CAD build for the part. Positions are in the model's coordinates, mm. A direction names the side the tool comes from. Give positions to 0.01 mm unless a question says otherwise; leave off trailing zeros. Order: outer loops, then holes, each group sorted by start corner. A loop starts at its lowest first (then second) coordinate and runs counter-clockwise, first axis right, second up. Notation, with made-up numbers: (9.25, 21.25) -> (67.25, 21.25) arc R20 cw to (67.25, 42.25) -> close; hole circle Ø4 at (-10, 76.25). An arc over 180 degrees is marked (long way). Answer as CSV lines item,"result".
```python
from build123d import *

# Parameters (mm, degrees)
SKETCH1_R            = 1.25
BOSS_EXTRUDE1_DEPTH  = 2.5
SKETCH3_W            = 12.5
SKETCH3_H            = 28.9
BOSS_EXTRUDE2_DEPTH  = 5.38
CUT_EXTRUDE1_DEPTH   = 9
LPATTERN1_COUNT      = 4
LPATTERN1_PITCH      = 10
LPATTERN1_COUNT_DIR2 = 2
LPATTERN1_PITCH_DIR2 = 10


with BuildPart() as part:
    # Sketch1 → Boss-Extrude1 (new body)
    with BuildSketch(Plane.XY):
        Polygon((9.79, -14.45), (-8.795857864, -14.45), (-10, -14.45), (-10, 14.45), (-9.79, 14.45), (8.795857864, 14.45), (10, 14.45), (10, -14.45), align=None)
        with Locations((-7.5, -5)):
            Circle(SKETCH1_R, mode=Mode.SUBTRACT)
        with Locations((-7.5, 5)):
            Circle(SKETCH1_R, mode=Mode.SUBTRACT)
        with Locations((7.5, 5)):
            Circle(SKETCH1_R, mode=Mode.SUBTRACT)
        with Locations((7.5, -5)):
            Circle(SKETCH1_R, mode=Mode.SUBTRACT)
    extrude(amount=BOSS_EXTRUDE1_DEPTH)

    # Sketch3 → Boss-Extrude2 (add)
    with BuildSketch(Plane.ZY.offset(10)):
        with Locations((-3.75, 0)):
            Rectangle(SKETCH3_W, SKETCH3_H)
    extrude(amount=BOSS_EXTRUDE2_DEPTH)

    # Sketch4 → Cut-Extrude1 (cut)
    with BuildSketch(Plane(origin=(0, 0, -10), x_dir=(-1, 0, 0), z_dir=(0, 0, -1))):
        with BuildLine():
            Line((13.62129958, 14.447528029), (13.62129958, 14.194772629))
            ThreePointArc((13.62129958, 14.194772629), (13.584011291, 14.095850288), (13.49070263, 14.046155824))
            ThreePointArc((13.49070263, 14.046155824), (13.278327951, 13.994947975), (13.081809662, 13.899523608))
            ThreePointArc((13.081809662, 13.899523608), (12.85675958, 13.447530026), (13.081809666, 12.995536447))
            ThreePointArc((13.081809666, 12.995536447), (13.278327608, 12.9001091), (13.490702635, 12.848898474))
            ThreePointArc((13.490702635, 12.848898474), (13.584017776, 12.799196632), (13.62129958, 12.700262029))
            Line((13.62129958, 12.700262029), (13.62129958, 12.194776629))
            ThreePointArc((13.62129958, 12.194776629), (13.584011291, 12.095854288), (13.49070263, 12.046159824))
            ThreePointArc((13.49070263, 12.046159824), (13.278327951, 11.994951975), (13.081809662, 11.899527608))
            ThreePointArc((13.081809662, 11.899527608), (12.85675958, 11.447534026), (13.081809666, 10.995540447))
            ThreePointArc((13.081809666, 10.995540447), (13.278327608, 10.9001131), (13.490702635, 10.848902474))
            ThreePointArc((13.490702635, 10.848902474), (13.584017776, 10.799200632), (13.62129958, 10.700266029))
            Line((13.62129958, 10.700266029), (13.62129958, 10.194780629))
            ThreePointArc((13.62129958, 10.194780629), (13.584011291, 10.095858288), (13.49070263, 10.046163824))
            ThreePointArc((13.49070263, 10.046163824), (13.278326417, 9.994943722), (13.081809662, 9.899506208))
            ThreePointArc((13.081809662, 9.899506208), (12.85675958, 9.447512626), (13.081809666, 8.995519047))
            ThreePointArc((13.081809666, 8.995519047), (13.278327608, 8.9000917), (13.490702635, 8.848881074))
            ThreePointArc((13.490702635, 8.848881074), (13.584009392, 8.799188772), (13.62129958, 8.700270029))
            Line((13.62129958, 8.700270029), (13.62129958, 8.194759229))
            ThreePointArc((13.62129958, 8.194759229), (13.584011291, 8.095836888), (13.49070263, 8.046142424))
            ThreePointArc((13.49070263, 8.046142424), (13.278327951, 7.994934575), (13.081809662, 7.899510208))
            ThreePointArc((13.081809662, 7.899510208), (12.85675958, 7.447516626), (13.081809666, 6.995523047))
            ThreePointArc((13.081809666, 6.995523047), (13.278327608, 6.9000957), (13.490702635, 6.848885074))
            ThreePointArc((13.490702635, 6.848885074), (13.584009392, 6.799192772), (13.62129958, 6.700274029))
            Line((13.62129958, 6.700274029), (13.62129958, 6.194763229))
            ThreePointArc((13.62129958, 6.194763229), (13.584011291, 6.095840888), (13.49070263, 6.046146424))
            ThreePointArc((13.49070263, 6.046146424), (13.278327951, 5.994938575), (13.081809662, 5.899514208))
            ThreePointArc((13.081809662, 5.899514208), (12.85675958, 5.447520626), (13.081809666, 4.995527047))
            ThreePointArc((13.081809666, 4.995527047), (13.278327608, 4.9000997), (13.490702635, 4.848889074))
            ThreePointArc((13.490702635, 4.848889074), (13.584009392, 4.799196772), (13.62129958, 4.700278029))
            Line((13.62129958, 4.700278029), (13.62129958, 4.447522629))
            Line((13.62129958, 4.447522629), (14.00229958, 4.447522629))
            Line((14.00229958, 4.447522629), (14.00229958, 14.447528029))
            Line((14.00229958, 14.447528029), (13.62129958, 14.447528029))
        make_face()
    cut_extrude1 = extrude(amount=-CUT_EXTRUDE1_DEPTH, mode=Mode.SUBTRACT)

    # LPattern1: Cut-Extrude1 4 × 2
    with Locations(*[Vector(0, -1, 0) * (i * LPATTERN1_PITCH) + Vector(0, 1, 0) * (j * LPATTERN1_PITCH_DIR2) for i in range(LPATTERN1_COUNT) for j in range(LPATTERN1_COUNT_DIR2) if (i, j) != (0, 0)]):
        add(cut_extrude1, mode=Mode.SUBTRACT)


solid = part.part
```
1) Pin check, flat tip, straight feed: P1, Ø7, axis at y = 6.5, z = -7.5, coming from the +X side. Stop position of the tip, or through.
Data:
P1,"stops at x = -10"
2) Which spindle directions (+Z, -Z, +X, -X, +Y, -Y) get a long thin tool onto all of the face, cutting with end or side? Do faces 5 (the cylindrical face through (-12.857, -6.545, -5.563)), 6 (the cylindrical face through (6.51, 4.24, 1.23)). Say none if no direction does.
Data:
face 5,"-Z"
face 6,"+Z, -Z"
3) Pull direction Y, two halves, no side cores. Call faces 1 (the flat face through (-13.8, 0.2, -1)), 2 (the cylindrical face through (6.51, -5.76, 1.23)), 3 (the flat face through (0, 0, 0)), 4 (the flat face through (-6.4, -14.45, 0.4)): pulls with the +Y half, pulls with the -Y half, needs draft (parallel to the pull), parting line crosses it, or undercut.
Data:
face 1,"undercut"
face 2,"undercut"
face 3,"needs draft"
face 4,"pulls with the -Y half"
4) Band-saw the part on A-A, the plane x = -7.5. Write the cut outline in (y, z), then the cut area to 4 significant figures.
Data:
outline,"(-14.45, 0) -> (-6.25, 0) -> (-6.25, 2.5) -> (-14.45, 2.5) -> close; (-3.75, 0) -> (3.75, 0) -> (3.75, 2.5) -> (-3.75, 2.5) -> close; (6.25, 0) -> (14.45, 0) -> (14.45, 2.5) -> (6.25, 2.5) -> close"
area,"59.75 mm2"
5) Band-saw the part on C-C, the plane x = 2. Write the cut outline in (y, z), then the cut area to 4 significant figures.
Data:
outline,"(-14.45, 0) -> (14.45, 0) -> (14.45, 2.5) -> (-14.45, 2.5) -> close"
area,"72.25 mm2"
6) Wall check: line 1 along X through (y, z) = (9.5, -5); line 2 along X through (y, z) = (-11, -7.5); line 3 along Z through (x, y) = (-0.5, -2.25). Give the ranges that are in metal, low to high. Write a range as [from, to].
Data:
line 1,"x = [-15.38, -14], [-12.86, -10]"
line 2,"x = [-15.38, -14], [-13.08, -10]"
line 3,"z = [0, 2.5]"
7) Band-saw the part on B-B, the plane y = 5.5. Write the cut outline in (x, z), then the cut area to 3 significant figures.
Data:
outline,"(-15.38, -10) -> (-14, -10) -> (-14, -1) -> (-12.86, -1) -> (-12.86, -10) -> (-10, -10) -> (-10, 0) -> (-8.65, 0) -> (-8.65, 2.5) -> (-15.38, 2.5) -> close; (-6.35, 0) -> (6.35, 0) -> (6.35, 2.5) -> (-6.35, 2.5) -> close; (8.65, 0) -> (10, 0) -> (10, 2.5) -> (8.65, 2.5) -> close"
area,"95.5 mm2"
